Part print with two shaded views. Sizes in mm from the minimum x, y, z corner. A direction names the side the tool comes from. Round coordinates to 2 decimals unless told otherwise and drop trailing zeros. Order: outer loops, then holes, each group sorted by start corner. A loop starts at its lowest first (then second) coordinate and runs counter-clockwise, first axis right, second up. Notation, with made-up numbers: M 34.5,-13.5 L 72.5,-13.5 A28 ccw 72.5,23.5 Z; hole C 76.5,50.25 d8. An arc over 180 degrees is marked long. Return JSON: item names as keys, results as strings. Group by question number.
Item 1: Slice it at C-C on x = 4. Write the cut outline in (y, z).
Item 2: Slice it at D-D on x = 2. Write the cut outline in (y, z), then the cut area to 3 significant figures.
Item 3: Probe line 1 along Y through (x, z) = (1.25, 4.3); line 2 along Y through (x, z) = (4.75, 3.5); line 3 along Z through (x, y) = (5, 20). List the from-to ranges inside material, lowest first.
Item 4: Pin check, flat tips, straight feed: pin 1 Ø1.7 at (x, z) = (4.5, 8) entering from +Y; pin 2 Ø1 at (x, y) = (5.5, 27.5) entering from +Z. Stop position of each tip, or through.
Item 5: Which spindle directions (+Z, -Z, +X, -X, +Y, -Y) get a long thin tool onto all of the face, cutting with end or side? Do the marked faces 1, 2 and 3. Say none if no direction does.
Item 6: Slice it at B-B on z = 4.3. Write the cut outline in (x, y), then the cut area to 3 significant figures.
Item 7: Slice it at A-A on y = 33.5. Write the cut outline in (x, z).
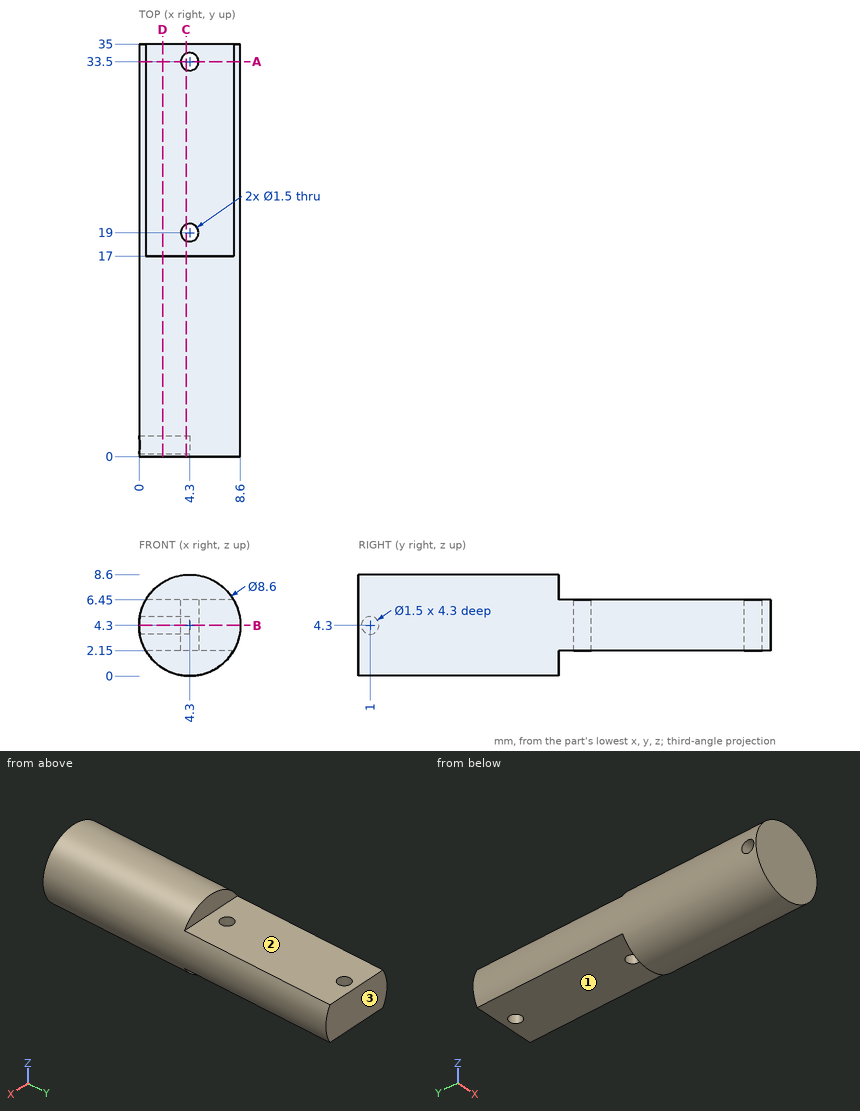
Output values:
{
 "1": {"outline": "M 0,0.01 L 17,0.01 L 17,2.15 L 18.31,2.15 L 18.31,6.45 L 17,6.45 L 17,8.59 L 0,8.59 Z; M 19.69,2.15 L 32.81,2.15 L 32.81,6.45 L 19.69,6.45 Z; M 34.19,2.15 L 35,2.15 L 35,6.45 L 34.19,6.45 Z; hole C 1,4.3 d1.5"},
 "2": {"outline": "M 0,0.67 L 17,0.67 L 17,2.15 L 35,2.15 L 35,6.45 L 17,6.45 L 17,7.93 L 0,7.93 Z; hole C 1,4.3 d1.5", "area": "199 mm²"},
 "3": {"line 1": "0 to 0.25, 1.75 to 35", "line 2": "0 to 18.4, 19.6 to 32.9, 34.1 to 35", "line 3": "2.15 to 6.45"},
 "4": {"pin 1": "y = 17", "pin 2": "z = 6.45"},
 "5": {"face 1": "-Z, +X, -X, +Y", "face 2": "+Z, +X, -X, +Y", "face 3": "+Z, -Z, +X, -X, +Y"},
 "6": {"outline": "M 0,0 L 8.6,0 L 8.6,35 L 0,35 L 0,1.75 L 4.3,1.75 L 4.3,0.25 L 0,0.25 Z; hole C 4.3,19 d1.5; hole C 4.3,33.5 d1.5", "area": "291 mm²"},
 "7": {"outline": "M 0.58,2.15 L 3.55,2.15 L 3.55,6.45 L 0.58,6.45 A4.3 ccw Z; M 5.05,2.15 L 8.02,2.15 A4.3 ccw 8.02,6.45 L 5.05,6.45 Z"}
}
